Could you check a few things on this model? Use its own coordinates, in mm. Face numbers are marked on the shaded views. Coordinates: 2 decimals unless noted, no trailing zeros. Write each loop counter-clockwise with the first axis right and the second up, starting at its lowest first coordinate (ties: lowest second). Pieces come first, ordered by that corner, then holes.
Item 1: If I drill on probe 1 along X at (y, z) = (0.25, 0.45); probe 2 along X at (y, z) = (1, -0.1); probe 3 along Y at (x, z) = (-3.25, 0.2), over which ranges is the centre line in solid material (lowest first)?
Item 2: I want a section at A-A on y = 4.75. Please give me the cut outline in (x, z).
Item 3: Thinking about a two-plate mould opening in X: for the marked faces 1, 2 and 3, which applies, +X half, -X half, draft (parallel to the pull), parting line (faces both ways), or undercut?
Item 4: I want a section at B-B on x = -3.25. Please give me the cut outline in (y, z), then the cut area to 3 significant figures.
from build123d import *

# Parameters (mm, degrees)
F1_DEPTH = 0.5
F2_R     = 0.25
F3_DEPTH = 10.9320678119


with BuildPart() as f1:
    # F0 (on Top) → F1 (new body, symmetric)
    with BuildSketch(Plane.XY):
        with BuildLine():
            Line((-3.00520382, 2.2980970389), (-4.9901862962, 0.3131145627))
            ThreePointArc((-4.9901862962, 0.3131145627), (-4.8244092491, -1.3134212566), (-4.1427869129, -2.7995207794))
            ThreePointArc((-4.1427869129, -2.7995207794), (-2.5428932188, -2.5428932188), (-2.7995207794, -4.1427869129))
            ThreePointArc((-2.7995207794, -4.1427869129), (-1.3134212566, -4.8244092491), (0.3131145627, -4.9901862962))
            Line((0.3131145627, -4.9901862962), (2.2980970389, -3.00520382))
            Line((2.2980970389, -3.00520382), (2.3758787848, -3.082985566))
            Line((2.3758787848, -3.082985566), (3.082985566, -2.3758787848))
            Line((3.082985566, -2.3758787848), (3.00520382, -2.2980970389))
            Line((3.00520382, -2.2980970389), (4.9901862962, -0.3131145627))
            ThreePointArc((4.9901862962, -0.3131145627), (4.8439927049, 1.2392476245), (4.2267303315, 2.6710954129))
            Line((4.2267303315, 2.6710954129), (4.0305086528, 2.4748737342))
            ThreePointArc((4.0305086528, 2.4748737342), (2.4748737342, 2.4748737342), (2.4748737342, 4.0305086528))
            Line((2.4748737342, 4.0305086528), (2.6710954129, 4.2267303315))
            ThreePointArc((2.6710954129, 4.2267303315), (1.2392476245, 4.8439927049), (-0.3131145627, 4.9901862962))
            Line((-0.3131145627, 4.9901862962), (-2.2980970389, 3.00520382))
            Line((-2.2980970389, 3.00520382), (-2.3758787848, 3.082985566))
            Line((-2.3758787848, 3.082985566), (-3.082985566, 2.3758787848))
            Line((-3.082985566, 2.3758787848), (-3.00520382, 2.2980970389))
        make_face()
    extrude(amount=F1_DEPTH, both=True)

    # F2 (on face) → F3 (cut, through all)
    with BuildSketch(Plane(origin=(2.7294321754, -2.7294321754, 0), x_dir=(0.7071067812, 0.7071067812, 0), z_dir=(0.7071067812, -0.7071067812, 0))):
        Circle(F2_R)
    extrude(amount=-F3_DEPTH, mode=Mode.SUBTRACT)


solid = f1.part
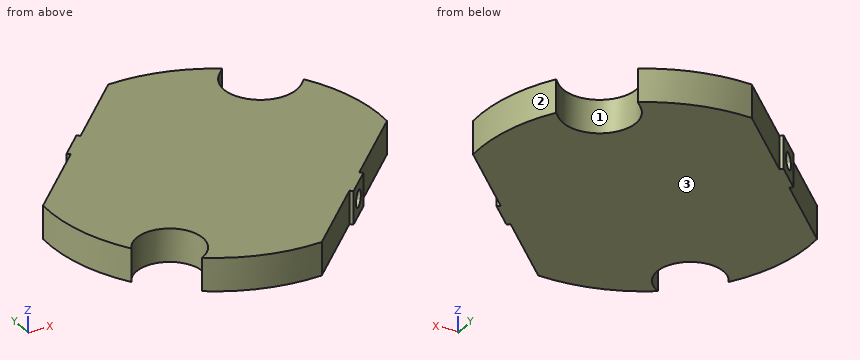
Response values:
1. probe 1: x = -4.99 to 4.99
1. probe 2: x = -4.3 to -1.32, -0.68 to 4.9
1. probe 3: y = -2.25 to 2.05
2. outline: (-0.55, -0.5) - (1.56, -0.5) - (1.56, 0.5) - (-0.55, 0.5) - close
3. face 1: undercut
3. face 2: +X half
3. face 3: draft
4. outline: (-2.25, -0.5) - (2.05, -0.5) - (2.05, 0.5) - (-2.25, 0.5) - close
4. area: 4.30 mm2
